Check sheet for the modelled part. Datum: model origin and axes. Units: mm. A direction names the side the tool comes from. Round coordinates to 2 decimals unless told otherwise and drop trailing zeros. Loops run counter-clockwise (first coordinate to the right, second up) from the corner with the lowest first, then second, coordinate; pieces in that order, holes last. Notation, with made-up numbers: (-34.75, -3) -> (-24.75, -3) arc R26 cw to (-24.75, 12) -> close; hole circle Ø6 at (-40, 40). An arc over 180 degrees is marked (long way). Return JSON: item names as keys, results as strings.
from build123d import *

# Parameters (mm, degrees)
SKETCH_1_R      = 1.6
EXTRUDE_1_DEPTH = 2
FILLET_2_R      = 2


with BuildPart() as part:
    # ｽｹｯﾁ1 → ﾎﾞｽ - 押し出し1 (new body)
    with BuildSketch(Plane.XY):
        Polygon((0, 0), (10, 0), (17.5, 0), (17.5, 10), (10, 10), (10, 30), (0, 30), align=None)
        with Locations((5, 25)):
            Circle(SKETCH_1_R, mode=Mode.SUBTRACT)
        with Locations(Location((5, 5, 0), (0, 0, 180))):
            Circle(SKETCH_1_R, mode=Mode.SUBTRACT)
        with Locations((13.75, 5)):
            Circle(SKETCH_1_R, mode=Mode.SUBTRACT)
    extrude(amount=EXTRUDE_1_DEPTH)

    # ﾌｨﾚｯﾄ2
    fillet_2_edges = [part.edges().sort_by_distance(p)[0] for p in [
        (0, 30, 1),
        (10, 30, 1),
        (10, 10, 1),
        (17.5, 10, 1),
        (17.5, 0, 1),
        (0, 0, 1),
    ]]
    fillet(fillet_2_edges, radius=FILLET_2_R)


solid = part.part
Q1. Tool access check on faces 1 (the flat face through (9, 0, 1)), 2 (the flat face through (10, 20, 1)). Record the directions out of +Z, -Z, +X, -X, +Y, -Y that give a thin tool (end or side, any length) a straight path to the whole face; none if there is none.
Results list:
{"face 1": "+Z, -Z, +X, -X, -Y", "face 2": "+Z, -Z, +X, +Y"}
Q2. Material ranges on line 1 (Y direction, x = 5, z = 1.55); line 2 (Y direction, x = 13.75, z = 1.2); line 3 (Y direction, x = 6, z = 0.7), recorded low to high.
Results list:
{"line 1": "0 to 3.4, 6.6 to 23.4, 26.6 to 30", "line 2": "0 to 3.4, 6.6 to 10", "line 3": "0 to 3.75, 6.25 to 23.75, 26.25 to 30"}
Q3. Go/stop test with flat-tipped pins: pin 1 (1 mm diameter, centred on y = 22.5, z = 0.5, fed in from +X); pin 2 (1.9 mm diameter, centred on x = 5, y = 5, fed in from +Z). Record where each tip stops, or that it passes through.
Results list:
{"pin 1": "x = 10", "pin 2": "through"}
Q4. Section check C-C (z = 1.45). Record the boundary of the cut face in (x, y), then the cut area to 3 significant figures.
Results list:
{"outline": "(0, 2) arc R2 ccw to (2, 0) -> (15.5, 0) arc R2 ccw to (17.5, 2) -> (17.5, 8) arc R2 ccw to (15.5, 10) -> (12, 10) arc R2 cw to (10, 12) -> (10, 28) arc R2 ccw to (8, 30) -> (2, 30) arc R2 ccw to (0, 28) -> close; hole circle Ø3.2 at (5, 5); hole circle Ø3.2 at (5, 25); hole circle Ø3.2 at (13.75, 5)", "area": "347 mm^2"}
Q5. Section check B-B (y = 5). Record the boundary of the cut face in (x, z).
Results list:
{"outline": "(0, 0) -> (3.4, 0) -> (3.4, 2) -> (0, 2) -> close; (6.6, 0) -> (12.15, 0) -> (12.15, 2) -> (6.6, 2) -> close; (15.35, 0) -> (17.5, 0) -> (17.5, 2) -> (15.35, 2) -> close"}
Q6. Section check A-A (x = 13.75). Record the boundary of the cut face in (y, z), then the cut area to 3 significant figures.
Results list:
{"outline": "(0, 0) -> (3.4, 0) -> (3.4, 2) -> (0, 2) -> close; (6.6, 0) -> (10, 0) -> (10, 2) -> (6.6, 2) -> close", "area": "13.6 mm^2"}
Q7. Draft check along X on faces 3 (the flat face through (14, 10, 1)), 4 (the cylindrical face through (3.73, 24.03, 0.99)), 5 (the cylindrical face through (0.57, 29.4, 1.01)). Enter one of: released by +X, released by -X, zero draft, split by the parting line, or undercut.
Results list:
{"face 3": "zero draft", "face 4": "undercut", "face 5": "released by -X"}
